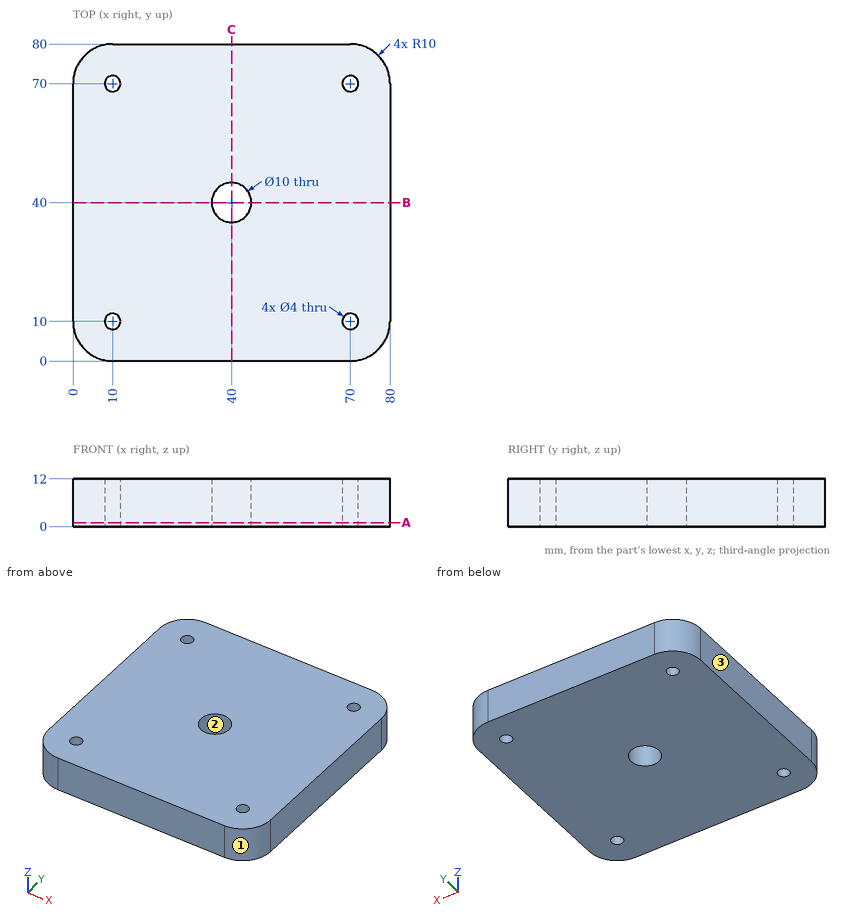
Input: dimensioned drawing with shaded views. Units: mm. Origin: part minimum x, y, z. Coordinates: 2 decimals unless noted, no trailing zeros. Order: outer loops, then holes, each group sorted by start corner. A loop starts at its lowest first (then second) coordinate and runs counter-clockwise, first axis right, second up. Notation, with made-up numbers: (-8.5, 49) - (30.5, 49) arc R14 ccw to (30.5, 75) - close; hole circle Ø7 at (-40, 11). An arc over 180 degrees is marked (long way). Return JSON: item names as keys, results as strings. Group by question number.
1. Cut plane B-B (y = 40). Output: boundary loops of the cut face in (x, z), plus the area to 3 significant figures.
2. Material intervals for line 1 along Y through (x, z) = (10, 8.5); line 2 along X through (y, z) = (70.5, 9); line 3 along X through (y, z) = (11.5, 1.5), sorted ascending. Write a range as [from, to].
3. Pin query (flat end, axial travel): pin 1 (1.5 mm diameter, centred on x = 8.5, z = 7, fed in from +Y); pin 2 (3 mm diameter, centred on x = 70, y = 70, fed in from +Z). Return the tip coordinate at first contact, or that it passes through.
4. Pull-direction query (X, two-part tool) for the marked faces 1, 2 and 3; classes: pulls with the +X half, pulls with the -X half, needs draft (parallel to the pull), parting line crosses it, or undercut.
5. Cut plane A-A (z = 1). Output: boundary loops of the cut face in (x, y), plus the area to 3 significant figures.
Resolved:
{
 "1": {"outline": "(0, 0) - (35, 0) - (35, 12) - (0, 12) - close; (45, 0) - (80, 0) - (80, 12) - (45, 12) - close", "area": "840 mm²"},
 "2": {"line 1": "y = [0, 8], [12, 68], [72, 80]", "line 2": "x = [0.01, 8.06], [11.94, 68.06], [71.94, 79.99]", "line 3": "x = [0, 8.68], [11.32, 68.68], [71.32, 80]"},
 "3": {"pin 1": "stops at y = 79.97", "pin 2": "passes through"},
 "4": {"face 1": "pulls with the +X half", "face 2": "undercut", "face 3": "pulls with the -X half"},
 "5": {"outline": "(0, 10) arc R10 ccw to (10, 0) - (70, 0) arc R10 ccw to (80, 10) - (80, 70) arc R10 ccw to (70, 80) - (10, 80) arc R10 ccw to (0, 70) - close; hole circle Ø4 at (10, 10); hole circle Ø4 at (10, 70); hole circle Ø10 at (40, 40); hole circle Ø4 at (70, 10); hole circle Ø4 at (70, 70)", "area": "6,190 mm²"}
}
